Verification items for the finished model (mm, model axes). Face numbers are marked on the shaded views. Coordinates: 2 decimals unless noted, no trailing zeros. Write each loop counter-clockwise with the first axis right and the second up, starting at its lowest first coordinate (ties: lowest second). Pieces come first, ordered by that corner, then holes. Notation, with made-up numbers: (-22, 46) -> (15, 46) arc R24 cw to (15, 78) -> close; hole circle Ø10 at (32, 78.5). An arc over 180 degrees is marked (long way). Use a Markdown table: item, result. Add a question column.
from build123d import *

# Parameters (mm, degrees)
SKETCH1_W           = 103
SKETCH1_H           = 83
BOSS_EXTRUDE1_DEPTH = 1.5
SKETCH2_W           = 103
SKETCH2_H           = 83
SKETCH2_W_2         = 100
SKETCH2_H_2         = 80
BOSS_EXTRUDE2_DEPTH = 35
SKETCH4_W           = 40
SKETCH4_H           = 35
CUT_EXTRUDE2_DEPTH  = 1.5
SKETCH5_W           = 5
SKETCH5_H           = 20
CUT_EXTRUDE3_DEPTH  = 1.5
SKETCH6_W           = 5
SKETCH6_H           = 20
CUT_EXTRUDE4_DEPTH  = 1.5
CUT_EXTRUDE5_DEPTH  = 2.5
SKETCH9_W           = 5
SKETCH9_H           = 20
CUT_EXTRUDE6_DEPTH  = 5


with BuildPart() as part:
    # Sketch1 → Boss-Extrude1 (new body)
    with BuildSketch(Plane(origin=(0, 0, 0), x_dir=(1, 0, 0), z_dir=(0, 1, 0))):
        with Locations((23.028301887, -29.825471698)):
            Rectangle(SKETCH1_W, SKETCH1_H)
    extrude(amount=BOSS_EXTRUDE1_DEPTH)

    # Sketch2 → Boss-Extrude2 (add)
    with BuildSketch(Plane(origin=(0, 1.5, 0), x_dir=(1, 0, 0), z_dir=(0, 1, 0))):
        with Locations((23.028301887, -29.825471698)):
            Rectangle(SKETCH2_W, SKETCH2_H)
        with Locations((23.028301887, -29.825471698)):
            Rectangle(SKETCH2_W_2, SKETCH2_H_2, mode=Mode.SUBTRACT)
    extrude(amount=BOSS_EXTRUDE2_DEPTH)

    # Sketch4 → Cut-Extrude2 (cut)
    with BuildSketch(Plane.ZY.offset(28.471698113)):
        with Locations((9.825471698, 19)):
            Rectangle(SKETCH4_W, SKETCH4_H)
    extrude(amount=-CUT_EXTRUDE2_DEPTH, mode=Mode.SUBTRACT)

    # Sketch5 → Cut-Extrude3 (cut)
    with BuildSketch(Plane.XY.offset(71.325471698)):
        with Locations((-4.471698113, 26.5)):
            Rectangle(SKETCH5_W, SKETCH5_H)
    extrude(amount=-CUT_EXTRUDE3_DEPTH, mode=Mode.SUBTRACT)

    # Sketch6 → Cut-Extrude4 (cut)
    with BuildSketch(Plane(origin=(74.528301887, 0, 0), x_dir=(0, 0, -1), z_dir=(1, 0, 0))):
        with Locations((-47.325471698, 26.5)):
            Rectangle(SKETCH6_W, SKETCH6_H)
    extrude(amount=-CUT_EXTRUDE4_DEPTH, mode=Mode.SUBTRACT)

    # Sketch7 → Cut-Extrude5 (cut, symmetric)
    with BuildSketch(Plane(origin=(23.028301887, 0, 0), x_dir=(0, 0, -1), z_dir=(1, 0, 0))):
        Polygon((-71.325471698, 28), (-69.825471698, 26.5), (-69.825471698, 25.5), (-71.325471698, 24), align=None)
        Polygon((11.674528302, 28), (11.674528302, 24), (10.174528302, 25.5), (10.174528302, 26.5), align=None)
    extrude(amount=CUT_EXTRUDE5_DEPTH, both=True, mode=Mode.SUBTRACT)

    # Sketch9 → Cut-Extrude6 (cut)
    with BuildSketch(Plane(origin=(0, 0, -11.674528302), x_dir=(-1, 0, 0), z_dir=(0, 0, -1))):
        with Locations((-50.528301887, 26.5)):
            Rectangle(SKETCH9_W, SKETCH9_H)
    extrude(amount=-CUT_EXTRUDE6_DEPTH, mode=Mode.SUBTRACT)


solid = part.part
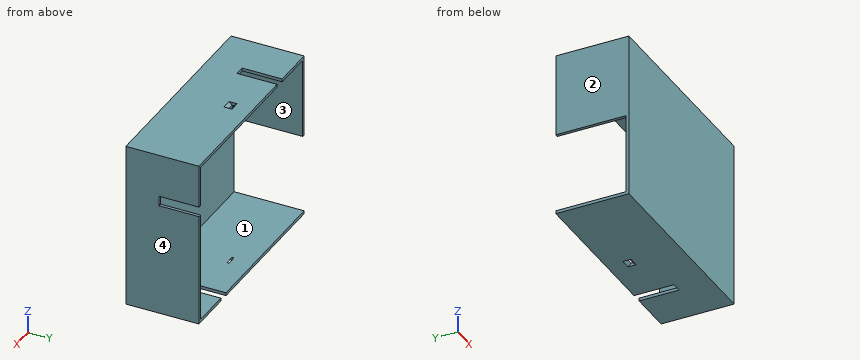
1) Release check for a two-part mould opening along X. For the marked faces 1, 2, 3 and 4 record: released by +X, released by -X, zero draft, split by the parting line, or undercut.
2) Cross-section at A-A on y = 18. Record the boundary of the cut face in (x, z).
3) Cross-section at D-D on z = 18. Record the boundary of the cut face in (x, y).
4) Gauge pin test, flat ends, axial feed: pin 1 (6 mm diameter, centred on x = 22, z = 21.5, fed in from +Y); pin 2 (8 mm diameter, centred on x = 25, z = 35, fed in from -Y); pin 3 (2 mm diameter, centred on y = 8, z = 4.5, fed in from -X); pin 4 (0.8 mm diameter, centred on x = -5.5, z = 70.5, fed in from +Y). Record the tip position at first contact, or that the pin passes through.
5) Cross-section at C-C on z = 63. Record the boundary of the cut face in (x, y), then the cut area to 4 significant figures.
6) Thickness scan on L1, parallel to Z at x = -7.5, y = 6; L2, parallel to X at y = 6.5, z = 58.5; L3, parallel to Y at x = 24, z = 36. Record the ranges inside material, lowest first.
7) Cross-section at B-B on x = 34. Record the boundary of the cut face in (y, z).
Returned:
| question | item | result |
|---|---|---|
| 1 | face 1 | zero draft |
| 1 | face 2 | released by -X |
| 1 | face 3 | undercut |
| 1 | face 4 | released by +X |
| 2 | outline | (-28.47, -11.67) -> (48.03, -11.67) -> (48.03, -10.17) -> (-28.47, -10.17) -> close; (-28.47, 29.83) -> (-26.97, 29.83) -> (-26.97, 69.83) -> (-6.97, 69.83) -> (-6.97, 71.33) -> (-28.47, 71.33) -> close; (-1.97, 69.83) -> (73.03, 69.83) -> (73.03, 49.83) -> (74.53, 49.83) -> (74.53, 71.33) -> (-1.97, 71.33) -> close; (53.03, -11.67) -> (74.53, -11.67) -> (74.53, 44.83) -> (73.03, 44.83) -> (73.03, -10.17) -> (53.03, -10.17) -> close |
| 3 | outline | (-28.47, 0) -> (74.53, 0) -> (74.53, 36.5) -> (73.03, 36.5) -> (73.03, 1.5) -> (-28.47, 1.5) -> close |
| 4 | pin 1 | stops at y = 1.5 |
| 4 | pin 2 | stops at y = 0 |
| 4 | pin 3 | stops at x = 73.03 |
| 4 | pin 4 | stops at y = 16.5 |
| 5 | outline | (-28.47, 0) -> (74.53, 0) -> (74.53, 36.5) -> (73.03, 36.5) -> (73.03, 1.5) -> (-26.97, 1.5) -> (-26.97, 36.5) -> (-28.47, 36.5) -> close |
| 5 | area | 259.5 mm² |
| 6 | L1 | z = -11.67 to -10.17, 69.83 to 71.33 |
| 6 | L2 | x = -28.47 to -26.97, 73.03 to 74.53 |
| 6 | L3 | y = 0 to 1.5 |
| 7 | outline | (0, -11.67) -> (36.5, -11.67) -> (36.5, -10.17) -> (1.5, -10.17) -> (1.5, 69.83) -> (36.5, 69.83) -> (36.5, 71.33) -> (0, 71.33) -> close |
